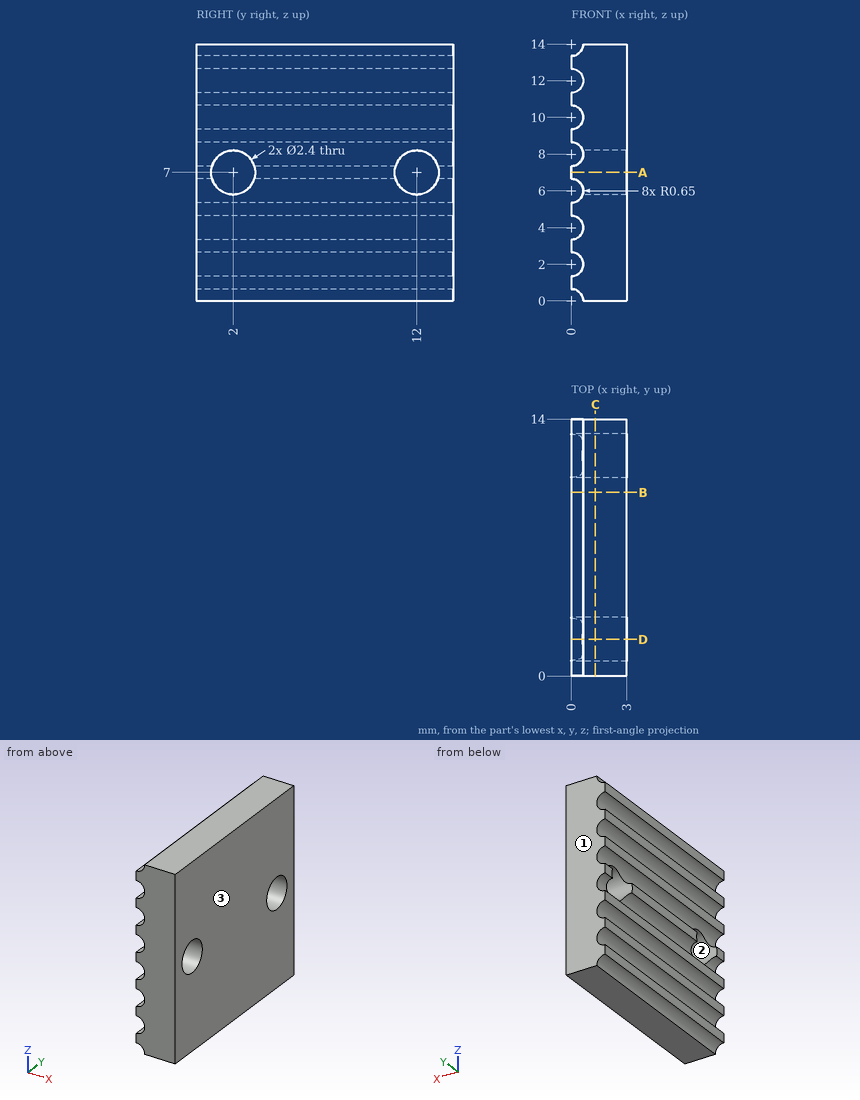
Drawing for the job (mm, zero at the part's lowest x, y, z). Coordinates: 2 decimals unless noted, no trailing zeros. Order: outer loops, then holes, each group sorted by start corner. A loop starts at its lowest first (then second) coordinate and runs counter-clockwise, first axis right, second up. Notation, with made-up numbers: (56, 45) -> (69, 45) arc R21 ccw to (69, 80) -> close; hole circle Ø11 at (16.5, -34). An arc over 180 degrees is marked (long way). Return JSON: item names as keys, results as strings.
Item 1: Pin check, flat tip, straight feed: P1, Ø2, axis at y = 2, z = 7, coming from the -X side. Stop position of the tip, or through.
Model answer:
{"P1": "passes through"}
Item 2: Wall check: line 1 along Y through (x, z) = (1.05, 7); line 2 along Y through (x, z) = (2, 6.25); line 3 along X through (y, z) = (1, 3.5). Give the ranges that are in metal, low to high. Write a range as from..to.
Model answer:
{"line 1": "y = 0..0.8, 3.2..10.8, 13.2..14", "line 2": "y = 0..1.06, 2.94..11.06, 12.94..14", "line 3": "x = 0.42..3"}
Item 3: Slice it at B-B (y = 10). Write the cut outline in (x, z), then the cut area to 3 significant figures.
Model answer:
{"outline": "(0, 0.65) arc R0.65 cw to (0.65, 0) -> (3, 0) -> (3, 14) -> (0.65, 14) arc R0.65 cw to (0, 13.35) -> (0, 12.65) arc R0.65 cw to (0, 11.35) -> (0, 10.65) arc R0.65 cw to (0, 9.35) -> (0, 8.65) arc R0.65 cw to (0, 7.35) -> (0, 6.65) arc R0.65 cw to (0, 5.35) -> (0, 4.65) arc R0.65 cw to (0, 3.35) -> (0, 2.65) arc R0.65 cw to (0, 1.35) -> close", "area": "37.4 mm²"}
Item 4: Slice it at C-C (x = 1.3). Write the cut outline in (y, z).
Model answer:
{"outline": "(0, 0) -> (14, 0) -> (14, 14) -> (0, 14) -> close; hole circle Ø2.4 at (2, 7); hole circle Ø2.4 at (12, 7)"}
Item 5: Mould opens along Y. For the marked faces 1, 2 and 3 say: pulls with the +Y half, pulls with the -Y half, needs draft (parallel to the pull), parting line crosses it, or undercut.
Model answer:
{"face 1": "pulls with the +Y half", "face 2": "undercut", "face 3": "needs draft"}
Item 6: Slice it at A-A (z = 7). Write the cut outline in (x, y), then the cut area to 3 significant figures.
Model answer:
{"outline": "(0, 0) -> (3, 0) -> (3, 0.8) -> (0, 0.8) -> close; (0, 3.2) -> (3, 3.2) -> (3, 10.8) -> (0, 10.8) -> close; (0, 13.2) -> (3, 13.2) -> (3, 14) -> (0, 14) -> close", "area": "27.6 mm²"}
Item 7: Slice it at D-D (y = 2). Write the cut outline in (x, z), then the cut area to 3 significant figures.
Model answer:
{"outline": "(0, 0.65) arc R0.65 cw to (0.65, 0) -> (3, 0) -> (3, 5.8) -> (0.62, 5.8) arc R0.65 cw to (0, 5.35) -> (0, 4.65) arc R0.65 cw to (0, 3.35) -> (0, 2.65) arc R0.65 cw to (0, 1.35) -> close; (0, 8.65) arc R0.65 cw to (0.62, 8.2) -> (3, 8.2) -> (3, 14) -> (0.65, 14) arc R0.65 cw to (0, 13.35) -> (0, 12.65) arc R0.65 cw to (0, 11.35) -> (0, 10.65) arc R0.65 cw to (0, 9.35) -> close", "area": "31.1 mm²"}
